```python
from build123d import *

# Parameters (mm, degrees)
SKETCH_1_W          = 97.6
SKETCH_1_H          = 97.6
SKETCH_1_R          = 1.59
EXTRUDE_1_DEPTH     = 2
SKETCH_2_R          = 1
CUT_EXTRUDE_1_DEPTH = 139.04173282
EXTRUDE_START       = -2
SKETCH_7_W          = 2.5
SKETCH_7_H          = 23.8
EXTRUDE_2_DEPTH     = 25
SKETCH_8_R          = 1.5
CUT_EXTRUDE_2_DEPTH = 141.273019501


with BuildPart() as part:
    # Эскиз1 → Бобышка-Вытянуть1 (new body)
    with BuildSketch(Plane(origin=(0, 0, 0), x_dir=(1, 0, 0), z_dir=(0, 1, 0))):
        with Locations((48.8, 48.8)):
            Rectangle(SKETCH_1_W, SKETCH_1_H)
        with Locations(Location((86.265001451, 91.665000306, 0), (0, 0, 270))):
            Circle(SKETCH_1_R, mode=Mode.SUBTRACT)
        with Locations(Location((88.805001451, 5.935000306, 0), (0, 0, 270))):
            Circle(SKETCH_1_R, mode=Mode.SUBTRACT)
        with Locations(Location((8.795001451, 5.935000306, 0), (0, 0, 270))):
            Circle(SKETCH_1_R, mode=Mode.SUBTRACT)
        with Locations(Location((12.605001451, 91.665000306, 0), (0, 0, 270))):
            Circle(SKETCH_1_R, mode=Mode.SUBTRACT)
        with BuildLine():
            Line((79.576520776, 92.6), (19.293482126, 92.6))
            ThreePointArc((19.293482126, 92.6), (17.512330868, 92.014021582), (16.426990408, 90.485000131))
            ThreePointArc((16.426990408, 90.485000131), (13.697675352, 87.817135476), (9.97357205, 88.652430089))
            ThreePointArc((9.97357205, 88.652430089), (6.759176917, 89.124368033), (5, 86.393002427))
            Line((5, 86.393002427), (5, 12.889708976))
            ThreePointArc((5, 12.889708976), (6.002770009, 10.651166513), (8.340714907, 9.909119546))
            ThreePointArc((8.340714907, 9.909119546), (10.982952752, 9.28356255), (12.616990516, 7.115000131))
            ThreePointArc((12.616990516, 7.115000131), (13.702330946, 5.5859785), (15.483482314, 5))
            Line((15.483482314, 5), (82.116520587, 5))
            ThreePointArc((82.116520587, 5), (83.897671955, 5.5859785), (84.983012386, 7.115000131))
            ThreePointArc((84.983012386, 7.115000131), (86.617049451, 9.283562094), (89.259286336, 9.909119736))
            ThreePointArc((89.259286336, 9.909119736), (91.597230458, 10.651167261), (92.6, 12.889709308))
            Line((92.6, 12.889709308), (92.6, 85.510507258))
            ThreePointArc((92.6, 85.510507258), (91.13495028, 88.088089), (88.170714907, 88.148147136))
            ThreePointArc((88.170714907, 88.148147136), (84.753959284, 87.961386993), (82.443012494, 90.485000131))
            ThreePointArc((82.443012494, 90.485000131), (81.357672034, 92.014021582), (79.576520776, 92.6))
        make_face(mode=Mode.SUBTRACT)
    extrude(amount=EXTRUDE_1_DEPTH)

    # Эскиз2 → Вырез-Вытянуть1 (cut, through all)
    with BuildSketch(Plane(origin=(0, 2, 0), x_dir=(1, 0, 0), z_dir=(0, 1, 0))):
        with Locations(Location((48.8, 95.1, 0), (0, 0, 270))):
            Circle(SKETCH_2_R)
    extrude(amount=-CUT_EXTRUDE_1_DEPTH, mode=Mode.SUBTRACT)

    # Эскиз7 → Бобышка-Вытянуть2 (add)
    with BuildSketch(Plane(origin=(0, 2, 0), x_dir=(1, 0, 0), z_dir=(0, 1, 0)).offset(EXTRUDE_START)):
        with Locations((1.25, 11.9)):
            Rectangle(SKETCH_7_W, SKETCH_7_H)
        with Locations((1.25, 85.7)):
            Rectangle(SKETCH_7_W, SKETCH_7_H)
        with Locations((96.35, 85.7)):
            Rectangle(SKETCH_7_W, SKETCH_7_H)
        with Locations((96.35, 11.9)):
            Rectangle(SKETCH_7_W, SKETCH_7_H)
    extrude(amount=-EXTRUDE_2_DEPTH)

    # Эскиз8 → Вырез-Вытянуть2 (cut, through all)
    with BuildSketch(Plane.ZY):
        with Locations((-80.630070031, -7.67342667)):
            Circle(SKETCH_8_R)
        with Locations(Location((-90.769929969, -17.32657333, 0), (0, 0, 180))):
            Circle(SKETCH_8_R)
        with Locations((-6.830070031, -17.32657333)):
            Circle(SKETCH_8_R)
        with Locations(Location((-16.969929969, -7.67342667, 0), (0, 0, 180))):
            Circle(SKETCH_8_R)
    extrude(amount=-CUT_EXTRUDE_2_DEPTH, mode=Mode.SUBTRACT)


solid = part.part
```
The listing builds one solid part. Answer for the finished solid, in the listing's coordinates (mm). A direction names the side the tool comes from. Give positions to 0.01 mm unless a question says otherwise; leave off trailing zeros. Order: outer loops, then holes, each group sorted by start corner. A loop starts at its lowest first (then second) coordinate and runs counter-clockwise, first axis right, second up. Notation, with made-up numbers: M -10,88 L 47,88 A19 ccw 47,101 Z; hole C 62,89.25 d4. An arc over 180 degrees is marked long. Put each result on its own line as item: value. Start each with the question number.
Item 1: The part is cut by section D-D, the plane z = -34. Determine the outline of the cut face in (x, y), and give its area (3 significant figures).
Item 2: The part is cut by section B-B, the plane z = -76.5. Determine the outline of the cut face in (x, y), and give its area (3 significant figures).
Item 3: A flat-ended cylindrical pin translates along its axis: P1, Ø4, axis at y = -7.67, z = -16.97, coming from the +X side. Find the tip coordinate at first contact, or state that the pin passes through.
Item 4: For a pull along Z with two mould halves and no side action, classify faces 5 (the face through (13.083, 0.986, -90.148)), 6 (the face through (97.6, 0.3, -48.1)), 7 (the face through (45, 1, 0)) as +Z half, -Z half, draft (parallel to the pull), parting line (faces both ways), or undercut.
Item 5: The part is cut by section C-C, the plane y = -4.75. Determine the outline of the cut face in (x, z).
Item 6: Find the intervals of material crossed by line 1 along X through (y, z) = (-12.25, -17); line 2 along Y through (x, z) = (4, -86.5), in increasing order.
Item 7: Which of the six approach directions +Z, -Z, +X, -X, +Y, -Y give full straight-line access (tool end or side, diameter ignored) to faces 1 (the face through (95.1, -12, -86)), 2 (the face through (13.681, 0.986, -5.602)), 3 (the face through (96, -12, -23.8)), 4 (the face through (1, -25, -12))?
Item 8: The part is cut by section A-A, the plane x = 62. Determine the outline of the cut face in (y, z).
Answer key:
1. outline: M 0,0 L 5,0 L 5,2 L 0,2 Z; M 92.6,0 L 97.6,0 L 97.6,2 L 92.6,2 Z
1. area: 20.0 mm²
2. outline: M 0,-25 L 2.5,-25 L 2.5,0 L 5,0 L 5,2 L 0,2 Z; M 92.6,0 L 95.1,0 L 95.1,-25 L 97.6,-25 L 97.6,2 L 92.6,2 Z
2. area: 145 mm²
3. P1: stops at x = 97.6
4. face 5: undercut
4. face 6: draft
4. face 7: +Z half
5. outline: M 0,-97.6 L 2.5,-97.6 L 2.5,-73.8 L 0,-73.8 Z; M 0,-23.8 L 2.5,-23.8 L 2.5,0 L 0,0 Z; M 95.1,-97.6 L 97.6,-97.6 L 97.6,-73.8 L 95.1,-73.8 Z; M 95.1,-23.8 L 97.6,-23.8 L 97.6,0 L 95.1,0 Z
6. line 1: x = 0 to 2.5, 95.1 to 97.6
6. line 2: y = 0 to 2
7. face 1: +Z, -Z, -Y
7. face 2: +Y, -Y
7. face 3: +X, -X, -Y
7. face 4: +Z, -Z, +X, -X, -Y
8. outline: M 0,-97.6 L 2,-97.6 L 2,-92.6 L 0,-92.6 Z; M 0,-5 L 2,-5 L 2,0 L 0,0 Z
